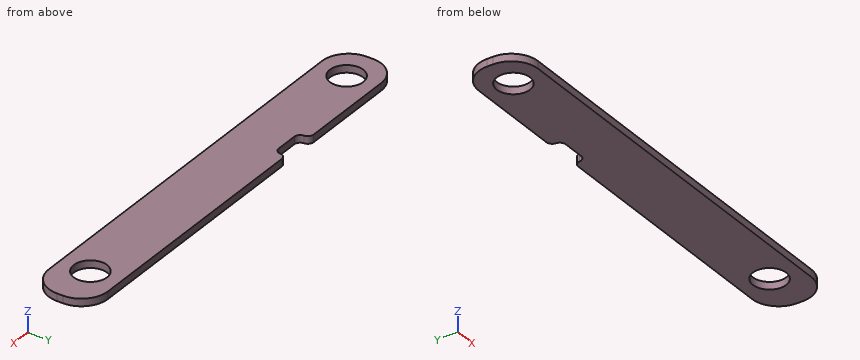
```python
from build123d import *

# Parameters (mm, degrees)
SKETCH2_W           = 381
SKETCH2_H           = 50.8
BOSS_EXTRUDE1_DEPTH = 6.35
SKETCH3_R           = 14.2875
SKETCH3_W           = 29.084677523
SKETCH3_H           = 9.575779023
CUT_EXTRUDE1_DEPTH  = 6.35
FILLET4_R           = 22.86
FILLET5_R           = 22.86
FILLET6_R           = 22.86
FILLET7_R           = 22.86
FILLET12_R          = 5.08
FILLET13_R          = 5.08
FILLET14_R          = 5.08
FILLET15_R          = 5.08


with BuildPart() as part:
    # Sketch2 → Boss-Extrude1 (new body)
    with BuildSketch(Plane.XY):
        with Locations((-46.726415094, 80.033962264)):
            Rectangle(SKETCH2_W, SKETCH2_H)
    extrude(amount=BOSS_EXTRUDE1_DEPTH)

    # Sketch3 → Cut-Extrude1 (cut)
    with BuildSketch(Plane.XY.offset(6.35)):
        with Locations((-208.27071376, 80.033962264)):
            Circle(SKETCH3_R)
        with Locations((106.195061698, 80.033962264)):
            Circle(SKETCH3_R)
        with Locations((-111.901475121, 100.646072753)):
            Rectangle(SKETCH3_W, SKETCH3_H)
    extrude(amount=-CUT_EXTRUDE1_DEPTH, mode=Mode.SUBTRACT)

    # Fillet4
    fillet4_edges = [part.edges().sort_by_distance(p)[0] for p in [
        (143.773584906, 105.433962264, 3.175),
    ]]
    fillet(fillet4_edges, radius=FILLET4_R)

    # Fillet5
    fillet5_edges = [part.edges().sort_by_distance(p)[0] for p in [
        (143.773584906, 54.633962264, 3.175),
    ]]
    fillet(fillet5_edges, radius=FILLET5_R)

    # Fillet6
    fillet6_edges = [part.edges().sort_by_distance(p)[0] for p in [
        (-237.226415094, 54.633962264, 3.175),
    ]]
    fillet(fillet6_edges, radius=FILLET6_R)

    # Fillet7
    fillet7_edges = [part.edges().sort_by_distance(p)[0] for p in [
        (-237.226415094, 105.433962264, 3.175),
    ]]
    fillet(fillet7_edges, radius=FILLET7_R)

    # Fillet12
    fillet12_edges = [part.edges().sort_by_distance(p)[0] for p in [
        (-126.443813883, 105.433962264, 3.175),
    ]]
    fillet(fillet12_edges, radius=FILLET12_R)

    # Fillet13
    fillet13_edges = [part.edges().sort_by_distance(p)[0] for p in [
        (-97.35913636, 105.433962264, 3.175),
    ]]
    fillet(fillet13_edges, radius=FILLET13_R)

    # Fillet14
    fillet14_edges = [part.edges().sort_by_distance(p)[0] for p in [
        (-126.443813883, 95.858183241, 3.175),
    ]]
    fillet(fillet14_edges, radius=FILLET14_R)

    # Fillet15
    fillet15_edges = [part.edges().sort_by_distance(p)[0] for p in [
        (-97.35913636, 95.858183241, 3.175),
    ]]
    fillet(fillet15_edges, radius=FILLET15_R)


solid = part.part
```
CAD build for the part. Positions are in the model's coordinates, mm. Round coordinates to 2 decimals unless told otherwise and drop trailing zeros. Write each loop counter-clockwise with the first axis right and the second up, starting at its lowest first coordinate (ties: lowest second). Pieces come first, ordered by that corner, then holes. Notation, with made-up numbers: (-17.75, 50) - (15.25, 50) arc R30 cw to (15.25, 74) - close; hole circle Ø8 at (-22, 61.25). An arc over 180 degrees is marked (long way). Return JSON: item names as keys, results as strings. Group by question number.
Item 1: Band-saw the part on B-B on x = -208. List the corners of the cut face in (y, z), plus the area to 3 significant figures.
Item 2: Probe probe 1 along X at (y, z) = (90, 5); probe 2 along X at (y, z) = (93, 5); probe 3 along Y at (x, z) = (121, 1.25). List the from-to ranges inside material, lowest first.
Item 3: Band-saw the part on D-D on z = 3.5. State how many separate pieces and enclosed holes the cut face has, plus the area to 3 significant figures.
Item 4: Band-saw the part on C-C on x = -109.5. List the corners of the cut face in (y, z), plus the area to 3 significant figures.
Item 5: Flat gauge pin, fed straight in: pin 1 Ø1.9 at (x, z) = (-109.5, 2.5) entering from +Y. Where does the tip first touch, or does it go through?
Item 6: Band-saw the part on A-A on y = 74. List the corners of the cut face in (x, z) (3 decimals), plus the area to 3 significant figures.
Resolved:
{
 "1": {"outline": "(54.63, 0) - (65.75, 0) - (65.75, 6.35) - (54.63, 6.35) - close; (94.32, 0) - (105.43, 0) - (105.43, 6.35) - (94.32, 6.35) - close", "area": "141 mm²"},
 "2": {"probe 1": "x = -235.99 to -218.51, -198.03 to 95.96, 116.43 to 142.53", "probe 2": "x = -234.71 to -214.27, -202.27 to 100.19, 112.2 to 141.26", "probe 3": "y = 54.63 to 105.43"},
 "3": {"separate pieces": "1", "enclosed holes": "2", "area": "17,300 mm²"},
 "4": {"outline": "(54.63, 0) - (95.86, 0) - (95.86, 6.35) - (54.63, 6.35) - close", "area": "262 mm²"},
 "5": {"pin 1": "stops at y = 95.86"},
 "6": {"outline": "(-236.958, 0) - (-221.222, 0) - (-221.222, 6.35) - (-236.958, 6.35) - close; (-195.32, 0) - (93.244, 0) - (93.244, 6.35) - (-195.32, 6.35) - close; (119.146, 0) - (143.505, 0) - (143.505, 6.35) - (119.146, 6.35) - close", "area": "2,090 mm²"}
}
